Job drawing, mm, ordinate dimensions from the low corner. One solid piece. A direction names the side the tool comes from. Round coordinates to 2 decimals unless told otherwise and drop trailing zeros. Loops run counter-clockwise (first coordinate to the right, second up) from the corner with the lowest first, then second, coordinate; pieces in that order, holes last.
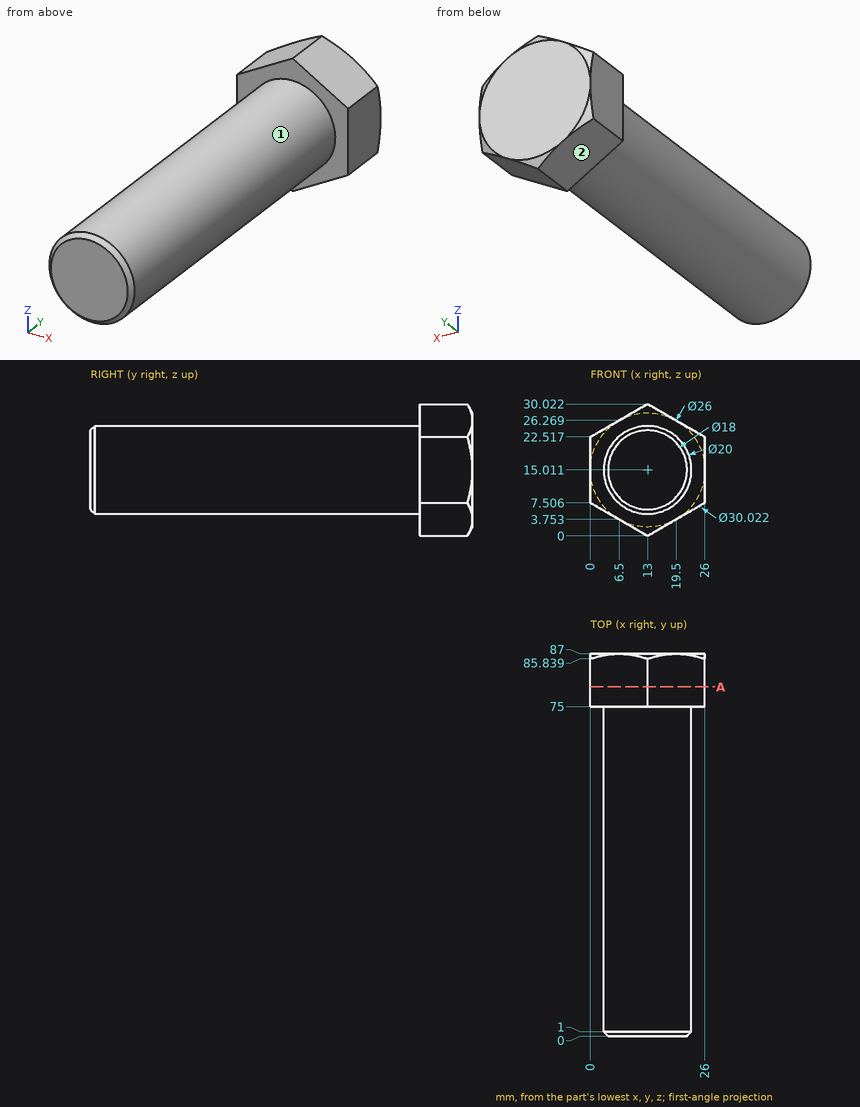
(1) Pin check, flat tips, straight feed: P1, Ø1, axis at y = 36, z = 10, coming from the -X side (1 decimal); P2, Ø3, axis at y = 74, z = 13.5, coming from the -X side; P3, Ø1, axis at x = 11, y = 50.5, coming from the +Z side; P4, Ø1, axis at x = 8, y = 55, coming from the -Z side. Stop position of each tip, or through.
Responses:
P1: stops at x = 4.1
P2: stops at x = 0
P3: stops at z = 24.9
P4: stops at z = 6.08
(2) Slice it at A-A on y = 79.5. List the corners of the cut face in (x, z) (1 decimal).
Responses:
outline: (0, 7.5) - (13, 0) - (26, 7.5) - (26, 22.5) - (13, 30) - (0, 22.5) - close
(3) Probe line 1 (Y direction, x = 10, z = 27.5); line 2 (Z direction, x = 13.25, y = 50) (1 decimal); line 3 (X direction, y = 52, z = 14.5). List the from-to ranges inside material, lowest first.
Responses:
line 1: y = 75 to 87
line 2: z = 5 to 25
line 3: x = 3.01 to 22.99
(4) Which spindle directions (+Z, -Z, +X, -X, +Y, -Y) get a long thin tool onto all of the face, cutting with end or side? Do the marked faces 1 and 2. Say none if no direction does.
Responses:
face 1: -Y
face 2: -Z, -X, +Y, -Y
